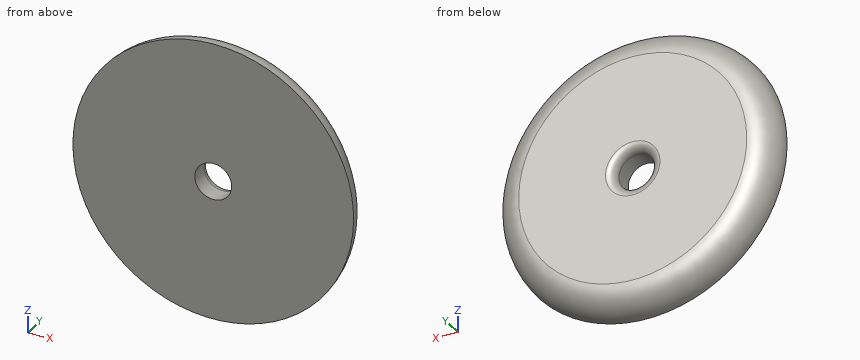
from build123d import *

# Parameters (mm, degrees)
SKETCH_1_R      = 16
SKETCH_1_R_2    = 2.1
EXTRUDE_1_DEPTH = 3
FILLET_1_R      = 3
FILLET_2_R      = 1


with BuildPart() as part:
    # Эскиз1 → Бобышка-Вытянуть1 (new body)
    with BuildSketch(Plane(origin=(0, 0, 0), x_dir=(1, 0, 0), z_dir=(0, 1, 0))):
        with Locations(Location((0, 0.566108198, 0), (0, 0, 270))):
            Circle(SKETCH_1_R)
        with Locations(Location((0, 0.566108198, 0), (0, 0, 270))):
            Circle(SKETCH_1_R_2, mode=Mode.SUBTRACT)
    extrude(amount=EXTRUDE_1_DEPTH)

    # Скругление1
    fillet_1_edges = [part.edges().sort_by_distance(p)[0] for p in [
        (0, 3, -16.566108198),
    ]]
    fillet(fillet_1_edges, radius=FILLET_1_R - 0.0001)  # a hair under: the kernel refuses the full size

    # Скругление2
    fillet_2_edges = [part.edges().sort_by_distance(p)[0] for p in [
        (0, 3, -2.666108198),
    ]]
    fillet(fillet_2_edges, radius=FILLET_2_R)


solid = part.part
The listing builds one solid part. Answer for the finished solid, in the listing's coordinates (mm). Coordinates: 2 decimals unless noted, no trailing zeros. Order: outer loops, then holes, each group sorted by start corner. A loop starts at its lowest first (then second) coordinate and runs counter-clockwise, first axis right, second up. Notation, with made-up numbers: (61, 39.5) -> (81, 39.5) arc R21 cw to (81, 65.5) -> close; hole circle Ø9 at (46, -3). An arc over 180 degrees is marked (long way). Answer in a Markdown table with one row per item. Add a question column.
Item 1: Find section B-B (y = 1.55). Write down the section's boundary in (x, z).
Item 2: This flat-tipped pin is pushed along its axis until it touches: P1, Ø1, axis at x = 10.5, y = 1, coming from the -Z side. Where does it stop, or does it pass through?
Item 3: Find the intervals of material crossed by L1, parallel to X at y = 1.55, z = 0; L2, parallel to X at y = 2.6, z = 1; L3, parallel to X at y = 1.85, z = 8, in increasing order. Write a range as from..to.
Result set:
| question | item | result |
|---|---|---|
| 1 | outline | circle Ø31.14 at (0, -0.57); hole circle Ø4.2 at (0, -0.57) |
| 2 | P1 | stops at z = -12.88 |
| 3 | L1 | x = -15.56..-2.02, 2.02..15.56 |
| 3 | L2 | x = -14.41..-1.68, 1.68..14.41 |
| 3 | L3 | x = -12.75..12.75 |
